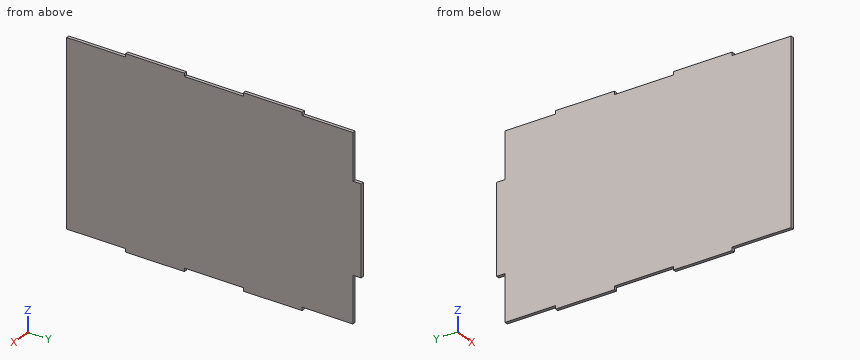
Autodesk Inventor part; units mm, degrees
ref_plane "YZ Plane" through (0, 0, 0) normal (1, 0, 0) x (0, 1, 0)
ref_plane "XZ Plane" through (0, 0, 0) normal (0, 1, 0) x (-1, 0, 0)
ref_plane "XY Plane" through (0, 0, 0) normal (0, 0, 1) x (1, 0, 0)
sketch "Sketch1" plane through (0, 0, 0) normal (1, 0, 0) x (0, 1, 0)
  line L0 (66.9402, 52.2533) -> (-113.0598, 52.2533)
  line L1 (-113.0598, 52.2533) -> (-113.0598, -61.7467)
  line L2 (-113.0598, -61.7467) -> (66.9402, -61.7467)
  line L3 (66.9402, -61.7467) -> (66.9402, 52.2533)
  point P0 (0, 0)
  dimension "d0" = 114
  dimension "d1" = 180
extrude "Extrusion1" add sketch "Sketch1" along normal blind 2
sketch "Sketch2" plane through (2, 0, 0) normal (1, 0, 0) x (0, 0, -1)
  line L0 (61.7467, 66.9402) -> (-52.2533, 66.9402)
  line L1 (-52.2533, 66.9402) -> (-22.2533, 66.9402)
  line L2 (-22.2533, 66.9402) -> (-22.2533, 61.9402)
  line L3 (-22.2533, 61.9402) -> (-52.2533, 61.9402)
  line L4 (-52.2533, 61.9402) -> (-52.2533, 66.9402)
  line L5 (61.7467, 66.9402) -> (31.7467, 66.9402)
  line L6 (31.7467, 66.9402) -> (31.7467, 61.9402)
  line L7 (31.7467, 61.9402) -> (61.7467, 61.9402)
  line L8 (61.7467, 61.9402) -> (61.7467, 66.9402)
  point P0 (0, 0)
  point P1 (31.7467, 66.9402)
  dimension "d4" = 30
  dimension "d5" = 30
  dimension "d6" = 5
extrude "Extrusion2" cut sketch "Sketch2" against normal blind 2
sketch "Sketch3" plane through (2, 0, 0) normal (1, 0, 0) x (0, 0, -1)
  line L0 (-52.2533, 61.9402) -> (-52.2533, -113.0598)
  line L1 (-52.2533, -113.0598) -> (-50.2533, -113.0598)
  line L2 (-50.2533, -113.0598) -> (-50.2533, -77.0598)
  line L3 (-50.2533, -77.0598) -> (-52.2533, -77.0598)
  line L4 (-52.2533, -77.0598) -> (-52.2533, -113.0598)
  line L5 (-52.2533, -41.0598) -> (-50.2533, -41.0598)
  line L6 (-50.2533, -41.0598) -> (-50.2533, -5.0598)
  line L7 (-50.2533, -5.0598) -> (-52.2533, -5.0598)
  line L8 (-52.2533, -5.0598) -> (-52.2533, -41.0598)
  line L9 (-52.2533, 61.9402) -> (-50.2533, 61.9402)
  line L10 (-50.2533, 61.9402) -> (-50.2533, 30.9402)
  line L11 (-50.2533, 30.9402) -> (-52.2533, 30.9402)
  line L12 (-52.2533, 30.9402) -> (-52.2533, 61.9402)
  line L13 (61.7467, 61.9402) -> (31.7467, 61.9402)
  line L14 (61.7467, 61.9402) -> (59.7467, 61.9402)
  line L15 (59.7467, 61.9402) -> (59.7467, 30.9402)
  line L16 (59.7467, 30.9402) -> (61.7467, 30.9402)
  line L17 (61.7467, 30.9402) -> (61.7467, 61.9402)
  line L18 (61.7467, -113.0598) -> (61.7467, 61.9402)
  line L19 (61.7467, -5.0598) -> (59.7467, -5.0598)
  line L20 (59.7467, -5.0598) -> (59.7467, -41.0598)
  line L21 (59.7467, -41.0598) -> (61.7467, -41.0598)
  line L22 (61.7467, -41.0598) -> (61.7467, -5.0598)
  line L23 (-52.2533, -113.0598) -> (61.7467, -113.0598)
  line L24 (61.7467, -77.0598) -> (59.7467, -77.0598)
  line L25 (59.7467, -77.0598) -> (59.7467, -113.0598)
  line L26 (59.7467, -113.0598) -> (61.7467, -113.0598)
  line L27 (61.7467, -113.0598) -> (61.7467, -77.0598)
  point P0 (0, 0)
  point P1 (60.7467, -77.0598)
  point P2 (60.7467, -41.0598)
  point P3 (60.7467, -5.0598)
  point P4 (60.7467, 30.9402)
  point P5 (61.7467, -41.0598)
  dimension "d9" = 2
  dimension "d10" = 2
  dimension "d11" = 36
  dimension "d12" = 36
  dimension "d13" = 36
  dimension "d14" = 36
  dimension "d15" = 36
extrude "Extrusion3" cut sketch "Sketch3" against normal blind 2
properties part number "inner_side"
Build history of the part. All positions in model axes, mm. Round coordinates to 2 decimals unless told otherwise and drop trailing zeros. Loops run counter-clockwise (first coordinate to the right, second up) from the corner with the lowest first, then second, coordinate; pieces in that order, holes last. Notation, with made-up numbers: (9, 10) -> (25, 10) arc R15 ccw to (25, 17) -> close; hole circle Ø1 at (27, -35.75). An arc over 180 degrees is marked (long way). Use CSV: the item, a comma, the result in double quotes. Start each with the question number.
Q1. Drill centre lines: L1, parallel to Z at x = 1.55, y = -14; L2, parallel to Y at x = 0.3, z = 32. Where is each one in solid material? Low to high.
Q2. Flat gauge pins, fed straight in: pin 1 Ø1.5 at (y, z) = (34.5, 27) entering from -X; pin 2 Ø0.6 at (x, z) = (1, 51.5) entering from +Y; pin 3 Ø0.6 at (x, z) = (0.5, -39) entering from +Y; pin 4 Ø1 at (x, y) = (1.5, -30) entering from +Z. Where does each tip first touch, or does it go through?
Q3. Saw through at B-B on y = -83.5. Give the cut face in (x, z), and give its area (3 significant figures).
Q4. Saw through at C-C on z = -48. Give the cut face in (x, y).
Q5. Saw through at A-A on x = 1.4. Give the cut face in (y, z), and give its area (3 significant figures).
Solutions:
1,L1,"z = -59.75 to 50.25"
1,L2,"y = -113.06 to 61.94"
2,pin 1,"stops at x = 0"
2,pin 2,"stops at y = 30.94"
2,pin 3,"stops at y = 61.94"
2,pin 4,"stops at z = 50.25"
3,outline,"(0, -59.75) -> (2, -59.75) -> (2, 50.25) -> (0, 50.25) -> close"
3,area,"220 mm^2"
4,outline,"(0, -113.06) -> (2, -113.06) -> (2, 61.94) -> (0, 61.94) -> close"
5,outline,"(-113.06, -59.75) -> (-77.06, -59.75) -> (-77.06, -61.75) -> (-41.06, -61.75) -> (-41.06, -59.75) -> (-5.06, -59.75) -> (-5.06, -61.75) -> (30.94, -61.75) -> (30.94, -59.75) -> (61.94, -59.75) -> (61.94, -31.75) -> (66.94, -31.75) -> (66.94, 22.25) -> (61.94, 22.25) -> (61.94, 50.25) -> (30.94, 50.25) -> (30.94, 52.25) -> (-5.06, 52.25) -> (-5.06, 50.25) -> (-41.06, 50.25) -> (-41.06, 52.25) -> (-77.06, 52.25) -> (-77.06, 50.25) -> (-113.06, 50.25) -> close"
5,area,"19,800 mm^2"
